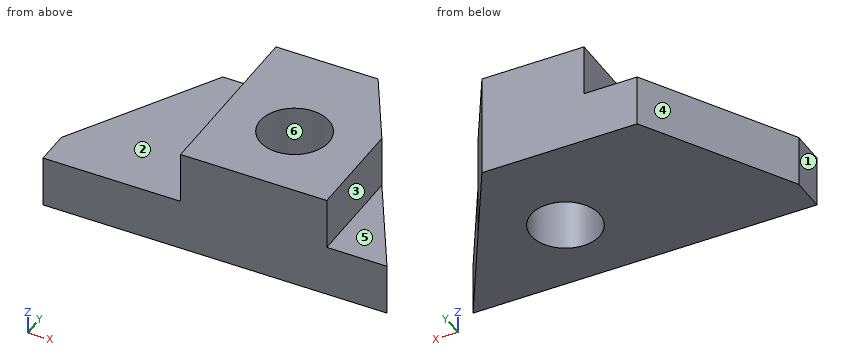
from build123d import *

# Parameters (mm, degrees)
BOSS_EXTRUDE1_DEPTH   = 19.05
BOSS_EXTRUDE1_2_DEPTH = 19.05
SKETCH1_3_R           = 12.7
BOSS_EXTRUDE2_DEPTH   = 38.1


with BuildPart() as part:
    # Sketch1 → Boss-Extrude1 (new body)
    with BuildSketch(Plane.XY):
        Polygon((-58.138751056, 66.675), (-89.301231836, 12.7), (-89.301231836, 0), (-38.501231836, 0), (-38.501231836, 66.675), align=None)
    extrude(amount=BOSS_EXTRUDE1_DEPTH)



with BuildPart() as body_2:
    # Sketch1 → Boss-Extrude1 2 (new body)
    with BuildSketch(Plane.XY):
        Polygon((15.473768164, 38.494829198), (15.473768164, 0), (37.698768164, 0), align=None)
    extrude(amount=BOSS_EXTRUDE1_2_DEPTH)


with BuildPart() as part_1:
    add(part.part)

    add(body_2.part)  # Boss-Extrude2 merges body 2
    # Sketch1<3> → Boss-Extrude2 (add)
    with BuildSketch(Plane.XY):
        Polygon((-38.501231836, 66.675), (-38.501231836, 0), (15.473768164, 0), (15.473768164, 38.494829198), (-0.796061034, 66.675), align=None)
        with Locations((-11.513731836, 28.575)):
            Circle(SKETCH1_3_R, mode=Mode.SUBTRACT)
    extrude(amount=BOSS_EXTRUDE2_DEPTH)


solid = part_1.part
CAD build for the part. Positions are in the model's coordinates, mm. Face numbers are marked on the shaded views. A direction names the side the tool comes from. Give positions to 0.01 mm unless a question says otherwise; leave off trailing zeros. Write each loop counter-clockwise with the first axis right and the second up, starting at its lowest first coordinate (ties: lowest second). Pieces come first, ordered by that corner, then holes. Notation, with made-up numbers: M -10,38 L 46,38 A25 ccw 46,59 Z; hole C 67,72 d6. An arc over 180 degrees is marked long. Put each result on its own line as item: value. Start each with the question number.
(1) Band-saw the part on B-B, the plane z = 16.5. Write the cut outline in (x, y) (3 decimals), and give its area (3 significant figures).
(2) Band-saw the part on D-D, the plane z = 22.5. Write the cut outline in (x, y) (3 decimals), and give its area (3 significant figures).
(3) Band-saw the part on A-A, the plane x = -3.5. Write the cut outline in (y, z) (3 decimals), and give its area (3 significant figures).
(4) Band-saw the part on C-C, the plane y = 49. Write the cut outline in (x, z), and give its area (3 significant figures).
(5) Mould opens along Y. For the marked faces 4, 5 and 6 say: +Y half, -Y half, draft (parallel to the pull), parting line (faces both ways), or undercut.
(6) Which spindle directions (+Z, -Z, +X, -X, +Y, -Y) get a long thin tool onto all of the face, cutting with end or side? Do the marked faces 1, 2 and 3. Say none if no direction does.
(7) Probe L1, parallel to X at y = 3, z = 35.5; L2, parallel to Z at x = -75, y = 9.5; L3, parallel to Y at x = -23, z = 12.5 (3 decimals). List the from-to ranges inside material, lowest first.
(8) Flat gauge pins, fed straight in: pin 1 Ø11 at (x, y) = (30.5, 15) entering from +Z; pin 2 Ø1 at (x, y) = (-34.5, 51) entering from -Z; pin 3 Ø10 at (y, z) = (8.5, 28) entering from -X; pin 4 Ø2 at (y, z) = (59.5, 24.5) entering from +X. Where does each tip first touch, or does it go through?
Response values:
1. outline: M -89.301,0 L 37.699,0 L -0.796,66.675 L -58.139,66.675 L -89.301,12.7 Z; hole C -11.514,28.575 d25.4
1. area: 5,840 mm2
2. outline: M -38.501,0 L 15.474,0 L 15.474,38.495 L -0.796,66.675 L -38.501,66.675 Z; hole C -11.514,28.575 d25.4
2. area: 2,860 mm2
3. outline: M 0,0 L 18.723,0 L 18.723,38.1 L 0,38.1 Z; M 38.427,0 L 66.675,0 L 66.675,38.1 L 38.427,38.1 Z
3. area: 1,790 mm2
4. outline: M -68.34,0 L 9.41,0 L 9.41,38.1 L -38.5,38.1 L -38.5,19.05 L -68.34,19.05 Z
4. area: 2,390 mm2
5. face 4: +Y half
5. face 5: draft
5. face 6: undercut
6. face 1: +Z, -Z, -X, +Y, -Y
6. face 2: +Z, -X, +Y, -Y
6. face 3: +Z, +X, +Y, -Y
7. L1: x = -38.5 to 15.47
7. L2: z = 0 to 19.05
7. L3: y = 0 to 23.157, 33.993 to 66.675
8. pin 1: stops at z = 19.05
8. pin 2: stops at z = 0
8. pin 3: stops at x = -38.5
8. pin 4: stops at x = 3.92
